Here's how the part is built. I have some questions about the finished solid (model axes, mm). A direction names the side the tool comes from. Give positions to 0.01 mm unless a question says otherwise; leave off trailing zeros. Loops run counter-clockwise (first coordinate to the right, second up) from the corner with the lowest first, then second, coordinate; pieces in that order, holes last. Notation, with made-up numbers: (35.25, 43.25) -> (54.25, 43.25) arc R24 ccw to (54.25, 72.25) -> close; hole circle Ø2 at (13.5, -10.5). An arc over 180 degrees is marked (long way). Answer in a Markdown table with one row per item. Add a question column.
Item 1: We'd pull the mould along X, two halves only. Please class faces 1 (the face through (2.67, -44.92, 2.96)), 2 (the face through (33.33, 8.17, 2.96)): released by +X, released by -X, zero draft, split by the parting line, or undercut.
Item 2: If we section it at A-A (x = -23): Write out the boundary of the cut face in (y, z).
Item 3: If we section it at D-D (z = 3.85): Give the number of separate pieces and of enclosed holes in the cut face, then the cut area to 3 significant figures.
Item 4: If we section it at B-B (x = -37): Write out the boundary of the cut face in (y, z).
Item 5: If I drill on line 1 (X direction, y = 16.5, z = 2.25); line 2 (Y direction, x = -23, z = 3.15); line 3 (Y direction, x = -24, z = 5.25), over which ranges is the centre line in solid material (lowest first)?
Item 6: If we section it at C-C (x = 0): Write out the boundary of the cut face in (y, z), then the cut area to 3 significant figures.
Item 7: For P1, Ø1.8, axis at y = -11, z = 3.5, coming from the +X side; P2, Ø1, axis at x = -30.5, z = 3.5, coming from the +Y side; P3, Ø3, axis at x = 8, z = 5.5, coming from the +Y side; P4, Ø13, axis at x = 0, y = 0, coming from the +Z side, each with a flat end and sliding along its axis, tell me the tip position at first contact or that it passes through.
Item 8: Which directions (+Z, -Z, +X, -X, +Y, -Y) give clear straight access to the entire face, cutting with the end or side of a thin tool? Please do faces 3 (the face through (36.946, -22, 2.958)), 4 (the face through (2.621, 30.557, 2.958)).
```python
from build123d import *

# Parameters (mm, degrees)
F0_R     = 11
F0_R_2   = 8
F1_DEPTH = 6


with BuildPart() as f1:
    # F0 (on Top) → F1 (new body)
    with BuildSketch(Plane.XY):
        with BuildLine():
            Line((39.030607, 18.044715), (41.415403, 22.174484))
            ThreePointArc((41.415403, 22.174484), (45.513832, 26.272208), (39.915627, 24.772689))
            Line((39.915627, 24.772689), (35.146743, 24.773099))
            ThreePointArc((35.146743, 24.773099), (0.003695, 43), (-35.142485, 24.779139))
            Line((-35.142485, 24.779139), (-39.911368, 24.779549))
            ThreePointArc((-39.911368, 24.779549), (-45.509316, 26.28003), (-41.411592, 22.181602))
            Line((-41.411592, 22.181602), (-39.027505, 18.051423))
            ThreePointArc((-39.027505, 18.051423), (-37.24094, -21.4968), (-3.888122, -42.823854))
            Line((-3.888122, -42.823854), (-1.504035, -46.954034))
            ThreePointArc((-1.504035, -46.954034), (-0.004516, -52.552239), (1.495965, -46.954291))
            Line((1.495965, -46.954291), (3.880762, -42.824522))
            ThreePointArc((3.880762, -42.824522), (37.237245, -21.5032), (39.030607, 18.044715))
        make_face()
        with BuildLine():
            Line((-14.234654, -24.899577), (-4.814016, -41.219841))
            ThreePointArc((-4.814016, -41.219841), (-35.941837, -20.746911), (-38.101611, 16.447409))
            Line((-38.101611, 16.447409), (-27.773521, -1.444918))
            Line((-27.773521, -1.444918), (-27.773521, -24.899577))
            Line((-27.773521, -24.899577), (-14.234654, -24.899577))
        make_face(mode=Mode.SUBTRACT)
        with Locations((-0.002148, -25)):
            Circle(F0_R, mode=Mode.SUBTRACT)
        Polygon((-15.765198, -22.248072), (-26.203172, -22.248072), (-26.203172, -4.165382), align=None, mode=Mode.SUBTRACT)
        with BuildLine():
            ThreePointArc((-11.652676, -1.509186), (0, -11.75), (11.652676, -1.509186))
            Line((11.652676, -1.509186), (12.40856, -1.509186))
            ThreePointArc((12.40856, -1.509186), (0, -12.5), (-12.40856, -1.509186))
            Line((-12.40856, -1.509186), (-11.652676, -1.509186))
        make_face(mode=Mode.SUBTRACT)
        with BuildLine():
            ThreePointArc((38.104437, 16.44086), (35.938271, -20.753088), (4.806931, -41.220667))
            Line((4.806931, -41.220667), (15.138096, -23.330116))
            Line((15.138096, -23.330116), (35.450427, -11.602786))
            Line((35.450427, -11.602786), (28.680994, 0.122216))
            Line((28.680994, 0.122216), (38.104437, 16.44086))
        make_face(mode=Mode.SUBTRACT)
        Polygon((27.149994, -2.529026), (32.368981, -11.568576), (16.708913, -20.609921), align=None, mode=Mode.SUBTRACT)
        Circle(F0_R_2, mode=Mode.SUBTRACT)
        with BuildLine():
            Line((12.40856, 1.509186), (11.652676, 1.509186))
            ThreePointArc((11.652676, 1.509186), (0, 11.75), (-11.652676, 1.509186))
            Line((-11.652676, 1.509186), (-12.40856, 1.509186))
            ThreePointArc((-12.40856, 1.509186), (0, 12.5), (12.40856, 1.509186))
        make_face(mode=Mode.SUBTRACT)
        with Locations((-21.649561, 12.50186)):
            Circle(F0_R, mode=Mode.SUBTRACT)
        Polygon((-11.384796, 24.777098), (-6.16581, 33.816648), (9.494259, 24.775304), align=None, mode=Mode.SUBTRACT)
        with BuildLine():
            ThreePointArc((-33.290421, 24.77898), (0.003566, 41.5), (33.294679, 24.773258))
            Line((33.294679, 24.773258), (12.635425, 24.775034))
            Line((12.635425, 24.775034), (-7.676906, 36.502363))
            Line((-7.676906, 36.502363), (-14.446339, 24.777361))
            Line((-14.446339, 24.777361), (-33.290421, 24.77898))
        make_face(mode=Mode.SUBTRACT)
        with Locations((21.651709, 12.498139)):
            Circle(F0_R, mode=Mode.SUBTRACT)
    extrude(amount=F1_DEPTH)


solid = f1.part
```
Recorded:
| question | item | result |
|---|---|---|
| 1 | face 1 | released by +X |
| 1 | face 2 | undercut |
| 2 | outline | (-36.33, 0) -> (-34.54, 0) -> (-34.54, 6) -> (-36.33, 6) -> close; (-24.9, 0) -> (-22.25, 0) -> (-22.25, 6) -> (-24.9, 6) -> close; (-9.71, 0) -> (1.59, 0) -> (1.59, 6) -> (-9.71, 6) -> close; (23.42, 0) -> (24.78, 0) -> (24.78, 6) -> (23.42, 6) -> close; (34.54, 0) -> (36.33, 0) -> (36.33, 6) -> (34.54, 6) -> close |
| 3 | separate pieces | 1 |
| 3 | enclosed holes | 12 |
| 3 | area | 2,420 mm^2 |
| 4 | outline | (-21.91, 0) -> (-18.79, 0) -> (-18.79, 6) -> (-21.91, 6) -> close; (14.54, 0) -> (24.78, 0) -> (24.78, 6) -> (14.54, 6) -> close |
| 5 | line 1 | x = -39.71 to -31.9, -11.4 to 11.41, 31.9 to 39.71 |
| 5 | line 2 | y = -36.33 to -34.54, -24.9 to -22.25, -9.71 to 1.59, 23.42 to 24.78, 34.54 to 36.33 |
| 5 | line 3 | y = -35.68 to -33.86, -24.9 to -22.25, -7.98 to 1.76, 23.25 to 24.78, 33.86 to 35.68 |
| 6 | outline | (-52.55, 0) -> (-36, 0) -> (-36, 6) -> (-52.55, 6) -> close; (-14, 0) -> (-12.5, 0) -> (-12.5, 6) -> (-14, 6) -> close; (-11.75, 0) -> (-8, 0) -> (-8, 6) -> (-11.75, 6) -> close; (8, 0) -> (11.75, 0) -> (11.75, 6) -> (8, 6) -> close; (12.5, 0) -> (24.78, 0) -> (24.78, 6) -> (12.5, 6) -> close; (30.26, 0) -> (32.07, 0) -> (32.07, 6) -> (30.26, 6) -> close; (41.5, 0) -> (43, 0) -> (43, 6) -> (41.5, 6) -> close |
| 6 | area | 247 mm^2 |
| 7 | P1 | stops at x = 41.8 |
| 7 | P2 | stops at y = 30.81 |
| 7 | P3 | stops at y = 42.51 |
| 7 | P4 | passes through |
| 8 | face 3 | +Z, -Z, +X |
| 8 | face 4 | +Z, -Z |
